The model under review builds one solid part; all positions refer to its coordinate system, in mm. A direction names the side the tool comes from. Give positions to 0.01 mm unless a question says otherwise; leave off trailing zeros. Order: outer loops, then holes, each group sorted by start corner. A loop starts at its lowest first (then second) coordinate and runs counter-clockwise, first axis right, second up. Notation, with made-up numbers: (73.5, -32) - (89.5, -32) arc R36 ccw to (89.5, 6) - close; hole circle Ø11 at (-9.5, -28.5). An arc over 180 degrees is marked (long way). Write item = value, one per line. Start each with the question number.
1. Machinability: for faces 4 (the cylindrical face through (-8.7, -23.22, -0.27)), 5 (the cylindrical face through (-57.1, 18.23, 1.13)), 6 (the flat face through (-90, 0, 0)), which of the approach directions +Z, -Z, +X, -X, +Y, -Y give a long, thin tool a straight path to every point of the face, cutting with its end or side? Answer none if there is none.
2. We need section A-A, the plane x = -9. Give the boundary of the cut face in (y, z), and give its area (3 significant figures).
3. We need section B-B, the plane z = -22. Give the boundary of the cut face in (x, y).
4. We need section D-D, the plane x = -72. Give the boundary of the cut face in (y, z), and give its area (3 significant figures).
5. Mouldability with a two-part tool opening along Y and no side actions: class faces 1 (the cylindrical face through (-1.48, 1.73, 7.81)), 2 (the cylindrical face through (-50.53, 16.12, 5.08)), 3 (the flat face through (-67, 3, 3)) as pulls with the +Y half, pulls with the -Y half, needs draft (parallel to the pull), parting line crosses it, or undercut.
6. We need section C-C, the plane x = -47.5. Give the boundary of the cut face in (y, z).
7. For P1, Ø5.5, axis at y = -10, z = -17.32, coming from the -X side; P2, Ø5, axis at y = 20, z = 0, coming from the +X side; P3, Ø3, axis at y = 22, z = 0, coming from the +X side; P4, Ø9, axis at y = -1.5, z = 2, coming from the +X side, all flat-tipped, find the tip position at first contact; note any pin that passes through.
8. Wall thickness on probe 1 along X at (y, z) = (-3, -8.5); probe 2 along Z at (x, y) = (-38.5, 0); probe 3 along Z at (x, y) = (-12.1, 0): over which ranges is each line inside the solid? List them lowest first.
from build123d import *

# Parameters (mm, degrees)
COQUE2_START                 = -56
COQUE2_OUTLINE_R             = 16.9
COQUE2_DEPTH                 = 43
COQUE2_START_2               = -59
COQUE2_2_OUTLINE_R           = 7
COQUE2_2_DEPTH               = 48
COQUE2_START_3               = -13
COQUE2_3_OUTLINE_R           = 11
COQUE2_3_OUTLINE_R_2         = 7
COQUE2_3_DEPTH               = 2
COQUE2_START_4               = -44.9
COQUE2_4_OUTLINE_R           = 17
COQUE2_4_OUTLINE_R_2         = 16.9
COQUE2_4_DEPTH               = 23.8
CHANFREIN1_SIZE              = 0.5
ESQUISSE6_R                  = 4
EXTRUSION1_DEPTH             = 10
ESQUISSE8_R                  = 4
EXTRUSION2_DEPTH             = 23
R_P_TITION_CIRCULAIRE1_COUNT = 6
CHANFREIN2_SIZE              = 0.5
EXTRUSION3_DEPTH             = 97.695398029
EXTRUSION3_DEPTH_BACK        = 97.695398029
ESQUISSE11_W                 = 21.903594892
ESQUISSE11_H                 = 3.021185502


# Read off the part's stored shape, not the designer's step: Coque2
with BuildPart() as part:
    # Esquisse1 → Base-Révolution (revolve)
    with BuildSketch(Plane.XY, mode=Mode.PRIVATE) as base_r_volution_sk:
        Polygon((-67, 0), (-67, 15), (-64, 15), (-64, 25), (-53, 25), (-53, 24.9), (-52.9, 24.9), (-52.9, 25), (-13.1, 25), (-13.1, 24.9), (-13, 24.9), (-13, 25), (-5, 25), (-5, 19), (-3, 19), (-3, 8), (0, 8), (0, 0), align=None)
    revolve(base_r_volution_sk.sketch.rotate(Axis((-92, 0, 0), (1, 0, 0)), 180), axis=Axis((-92, 0, 0), (1, 0, 0)))

    # Coque2 outline → Coque2 (cut)
    with BuildSketch(Plane.YZ.offset(COQUE2_START)):
        Circle(COQUE2_OUTLINE_R)
    extrude(amount=COQUE2_DEPTH, mode=Mode.SUBTRACT)

    # Coque2 2 outline → Coque2 2 (cut)
    with BuildSketch(Plane.YZ.offset(COQUE2_START_2)):
        Circle(COQUE2_2_OUTLINE_R)
    extrude(amount=COQUE2_2_DEPTH, mode=Mode.SUBTRACT)

    # Coque2 3 outline → Coque2 3 (cut)
    with BuildSketch(Plane.YZ.offset(COQUE2_START_3)):
        Circle(COQUE2_3_OUTLINE_R)
        Circle(COQUE2_3_OUTLINE_R_2, mode=Mode.SUBTRACT)
    extrude(amount=COQUE2_3_DEPTH, mode=Mode.SUBTRACT)

    # Coque2 4 outline → Coque2 4 (cut)
    with BuildSketch(Plane.YZ.offset(COQUE2_START_4)):
        Circle(COQUE2_4_OUTLINE_R)
        Circle(COQUE2_4_OUTLINE_R_2, mode=Mode.SUBTRACT)
    extrude(amount=COQUE2_4_DEPTH, mode=Mode.SUBTRACT)

    # Esquisse4 → Trou taraudé M5x0.81 (revolve, cut)
    with BuildSketch(Plane(origin=(-64, 20, 0), x_dir=(0, 0, 1), z_dir=(0, 1, 0))):
        Polygon((0, 0), (0, 15.212435565), (2.1, 14), (2.1, 0), align=None)
    trou_taraud_m5x0_81 = revolve(axis=Axis((-70.35, 20, 0), (1, 0, 0)), mode=Mode.SUBTRACT)

    # Chanfrein1
    chanfrein1_edges = [part.edges().sort_by_distance(p)[0] for p in [
        (-67, 15, 0),
    ]]
    chamfer(chanfrein1_edges, length=CHANFREIN1_SIZE)

    # Esquisse6 → Extrusion1 (cut)
    with BuildSketch(Plane(origin=(0, 0, 0), x_dir=(0, 0, -1), z_dir=(1, 0, 0))):
        with Locations(Location((0, 0, 0), (0, 0, 90))):
            Circle(ESQUISSE6_R)
    extrude(amount=-EXTRUSION1_DEPTH, mode=Mode.SUBTRACT)

    # Esquisse8 → Extrusion2 (add)
    with BuildSketch(Plane.ZY.offset(67)):
        with Locations(Location((0, 0, 0), (0, 0, 90))):
            Circle(ESQUISSE8_R)
    extrude(amount=EXTRUSION2_DEPTH)

    # Esquisse9 → Trou taraudé M31 (revolve, cut)
    with BuildSketch(Plane(origin=(-5, 22, 0), x_dir=(0, 0, -1), z_dir=(0, 1, 0))):
        Polygon((0, 0), (0, 8.251075774), (1.25, 7.5), (1.25, 0), align=None)
    trou_taraud_m31 = revolve(axis=Axis((1.35, 22, 0), (-1, 0, 0)), mode=Mode.SUBTRACT)

    # Répétition circulaire1: Trou taraudé M5x0.81, Trou taraudé M31 ×6 about axis
    r_p_tition_circulaire1_axis = Axis((0, 0, 0), (1, 0, 0))
    add([trou_taraud_m5x0_81.rotate(r_p_tition_circulaire1_axis, i * 360 / R_P_TITION_CIRCULAIRE1_COUNT) for i in range(1, R_P_TITION_CIRCULAIRE1_COUNT)], mode=Mode.SUBTRACT)
    add([trou_taraud_m31.rotate(r_p_tition_circulaire1_axis, i * 360 / R_P_TITION_CIRCULAIRE1_COUNT) for i in range(1, R_P_TITION_CIRCULAIRE1_COUNT)], mode=Mode.SUBTRACT)

    # Chanfrein2
    chanfrein2_edges = [part.edges().sort_by_distance(p)[0] for p in [
        (-90, -4, 0),
    ]]
    chamfer(chanfrein2_edges, length=CHANFREIN2_SIZE)

    # Esquisse11 → Extrusion3 (cut, two sides: drawn at the far end of the back side and taken through both)
    with BuildSketch(Plane.XY.offset(-EXTRUSION3_DEPTH_BACK)):
        with Locations((-80.650230715, 4.710592751)):
            Rectangle(ESQUISSE11_W, ESQUISSE11_H)
    extrude(amount=EXTRUSION3_DEPTH + EXTRUSION3_DEPTH_BACK, mode=Mode.SUBTRACT)


solid = part.part
Model answer:
q1.face_4 = +X
q1.face_5 = -X
q1.face_6 = +Z, -Z, -X, +Y, -Y
q2.outline = circle Ø50 at (0, 0); hole circle Ø2.5 at (-22, 0); hole circle Ø2.5 at (-11, -19.05); hole circle Ø2.5 at (-11, 19.05); hole circle Ø8 at (0, 0); hole circle Ø2.5 at (11, -19.05); hole circle Ø2.5 at (11, 19.05); hole circle Ø2.5 at (22, 0)
q2.area = 1,880 mm2
q3.outline = (-64, -11.87) - (-53, -11.87) - (-53, -11.66) - (-52.9, -11.66) - (-52.9, -11.87) - (-13.1, -11.87) - (-13.1, -11.66) - (-13, -11.66) - (-13, -11.87) - (-5, -11.87) - (-5, 11.87) - (-13, 11.87) - (-13, 11.66) - (-13.1, 11.66) - (-13.1, 11.87) - (-52.9, 11.87) - (-52.9, 11.66) - (-53, 11.66) - (-53, 11.87) - (-64, 11.87) - close
q4.outline = (3.2, -2.4) - (3.2, 2.4) arc R4 ccw (long way) to start
q4.area = 47.6 mm2
q5.face_1 = parting line crosses it
q5.face_2 = undercut
q5.face_3 = needs draft
q6.outline = circle Ø50 at (0, 0); hole circle Ø33.8 at (0, 0)
q7.P1 = -64
q7.P2 = -3
q7.P3 = -5
q7.P4 = 0
q8.probe_1 = -67 to -56, -11 to -3
q8.probe_2 = -25 to -17, 17 to 25
q8.probe_3 = -25 to -11, 11 to 25
